Verification items for this drawing (mm, ordinates from the low corner). A direction names the side the tool comes from. Round coordinates to 2 decimals unless told otherwise and drop trailing zeros. Write each loop counter-clockwise with the first axis right and the second up, starting at its lowest first coordinate (ties: lowest second). Pieces come first, ordered by that corner, then holes. Notation, with made-up numbers: (9.25, -37) -> (52.25, -37) arc R25 cw to (52.25, -19) -> close; hole circle Ø8 at (24.25, 43). An arc over 180 degrees is marked (long way). One line per item, written item: value.
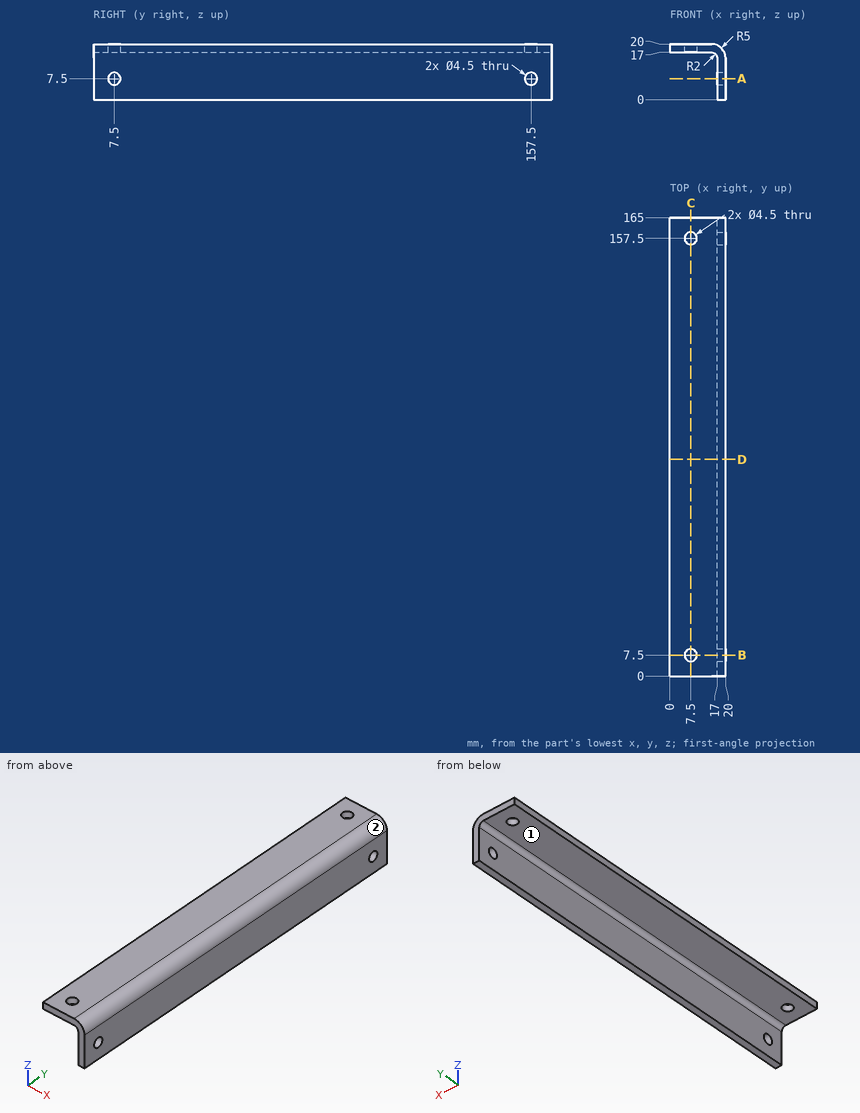
Item 1: Material ranges on line 1 along Y through (x, z) = (19, 7.5); line 2 along Z through (x, y) = (13.75, 55), recorded low to high.
Result set:
line 1: 0 to 5.25, 9.75 to 155.25, 159.75 to 165
line 2: 17 to 20
Item 2: Depth check by flat-ended pin: pin 1 (4.5 mm diameter, centred on x = 8, y = 42, fed in from -Z); pin 2 (5 mm diameter, centred on y = 7.5, z = 7.5, fed in from -X); pin 3 (3.5 mm diameter, centred on y = 157.5, z = 7.5, fed in from +X). Enter the tip coordinate at first touch or a pass-through.
Result set:
pin 1: z = 17
pin 2: x = 17
pin 3: through
Item 3: Sectioned sample at C-C (x = 7.5). Enter the section's corners in (y, z), then the cut area to 3 significant figures.
Result set:
outline: (0, 17) -> (5.25, 17) -> (5.25, 20) -> (0, 20) -> close; (9.75, 17) -> (155.25, 17) -> (155.25, 20) -> (9.75, 20) -> close; (159.75, 17) -> (165, 17) -> (165, 20) -> (159.75, 20) -> close
area: 468 mm^2
Item 4: Sectioned sample at B-B (y = 7.5). Enter the section's corners in (x, z).
Result set:
outline: (0, 17) -> (5.25, 17) -> (5.25, 20) -> (0, 20) -> close; (9.75, 17) -> (15, 17) arc R2 cw to (17, 15) -> (17, 9.75) -> (20, 9.75) -> (20, 15) arc R5 ccw to (15, 20) -> (9.75, 20) -> close; (17, 0) -> (20, 0) -> (20, 5.25) -> (17, 5.25) -> close
Item 5: Sectioned sample at A-A (z = 7.5). Enter the section's corners in (x, y).
Result set:
outline: (17, 0) -> (20, 0) -> (20, 5.25) -> (17, 5.25) -> close; (17, 9.75) -> (20, 9.75) -> (20, 155.25) -> (17, 155.25) -> close; (17, 159.75) -> (20, 159.75) -> (20, 165) -> (17, 165) -> close
Item 6: Tool access check on the marked faces 1 and 2. Record the directions out of +Z, -Z, +X, -X, +Y, -Y that give a thin tool (end or side, any length) a straight path to the whole face; none if there is none.
Result set:
face 1: -Z, -X, +Y, -Y
face 2: +Z, +X, +Y, -Y
Item 7: Sectioned sample at D-D (y = 78). Enter the section's corners in (x, z), then the cut area to 3 significant figures.
Result set:
outline: (0, 17) -> (15, 17) arc R2 cw to (17, 15) -> (17, 0) -> (20, 0) -> (20, 15) arc R5 ccw to (15, 20) -> (0, 20) -> close
area: 106 mm^2
